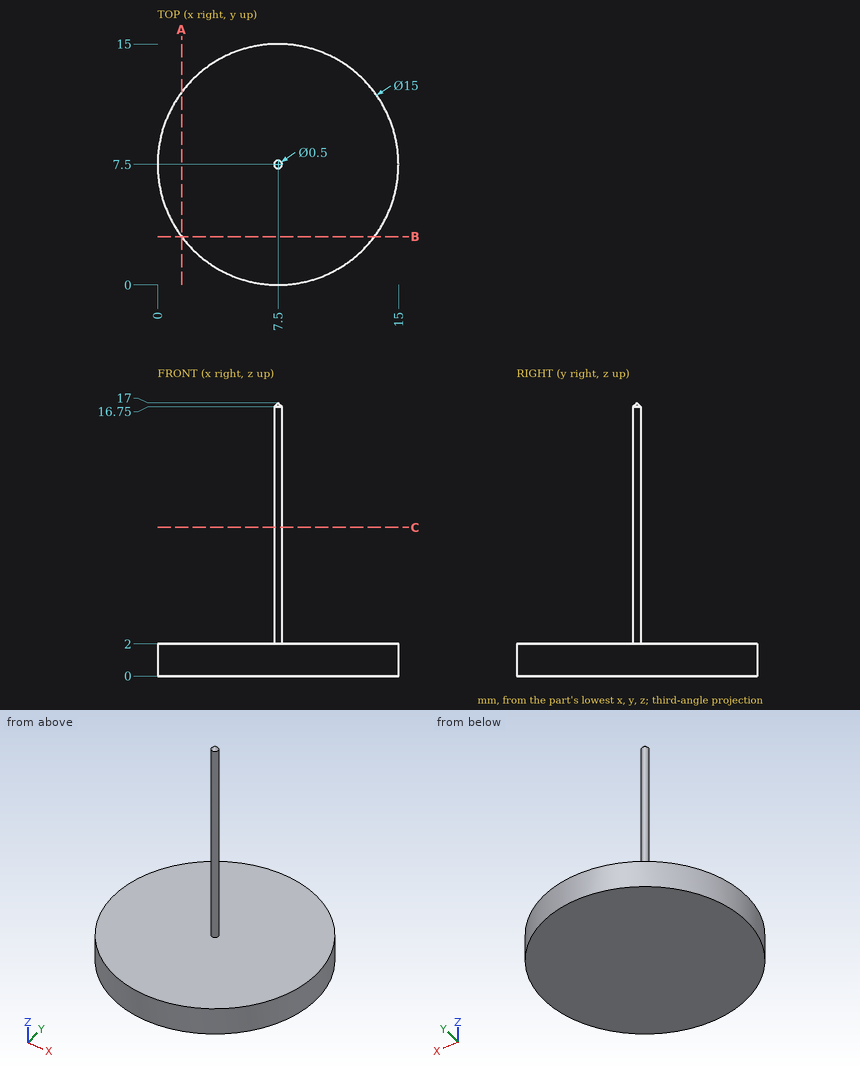
Here's the drawing with two shaded views (mm, measured from the low corner). I have some questions. Coordinates: 2 decimals unless noted, no trailing zeros. Write each loop counter-clockwise with the first axis right and the second up, starting at its lowest first coordinate (ties: lowest second). Pieces come first, ordered by that corner, then holes. Notation, with made-up numbers: M 88.25,-16.75 L 115.25,-16.75 A21 cw 115.25,9.25 Z; hole C -28.5,56 d11. An arc over 180 degrees is marked long. Write item = value, one per line. Start each with the question number.
Q1. I'm going to push flat-ended pins straight in: pin 1 (3 mm diameter, centred on y = 4, z = 2, fed in from +X); pin 2 (8 mm diameter, centred on x = 8, z = 11, fed in from -Y); pin 3 (4.5 mm diameter, centred on x = 5, y = 8, fed in from +Z). Where does each tip first touch, or does it pass through?
Q2. If we section it at C-C, the plane z = 9.25: Write out the boundary of the cut face in (x, y).
Q3. If we section it at B-B, the plane y = 3: Write out the boundary of the cut face in (x, z).
Q4. If I drill on L1, parallel to Z at x = 14, y = 4.5; L2, parallel to Y at x = 7.5, z = 6; L3, parallel to X at y = 9.25, z = 1.5, over which ranges is the centre line in solid material (lowest first)? Write a range as [from, to].
Q5. If we section it at A-A, the plane x = 1.5: Write out the boundary of the cut face in (y, z).
Check sheet entries:
q1.pin_1 = 14.73
q1.pin_2 = 7.25
q1.pin_3 = 2
q2.outline = C 7.5,7.5 d0.5
q3.outline = M 1.5,0 L 13.5,0 L 13.5,2 L 1.5,2 Z
q4.L1 = [0, 2]
q4.L2 = [7.25, 7.75]
q4.L3 = [0.21, 14.79]
q5.outline = M 3,0 L 12,0 L 12,2 L 3,2 Z
